```python
from build123d import *

# Parameters (mm, degrees)
F0_W     = 183.4
F0_H     = 218.4
F1_DEPTH = 49.6
F2_T     = -1.2
F3_R     = 2
F4_R     = 0.8


with BuildPart() as f1:
    # F0 (on Top) → F1 (new body)
    with BuildSketch(Plane.XY):
        Rectangle(F0_W, F0_H)
    extrude(amount=F1_DEPTH)

    # F2
    f2_openings = [f1.faces().sort_by_distance(p)[0] for p in [
        (0, 0, 0),
    ]]
    offset(amount=F2_T, openings=f2_openings)

    # F3
    f3_edges = [f1.edges().sort_by_distance(p)[0] for p in [
        (-91.7, -109.2, 24.8),
        (-91.7, 109.2, 24.8),
        (91.7, 109.2, 24.8),
        (91.7, -109.2, 24.8),
    ]]
    fillet(f3_edges, radius=F3_R)

    # F4
    f4_edges = [f1.edges().sort_by_distance(p)[0] for p in [
        (-90.5, -108, 24.2),
        (90.5, -108, 24.2),
        (90.5, 108, 24.2),
        (-90.5, 108, 24.2),
    ]]
    fillet(f4_edges, radius=F4_R)


solid = f1.part
```
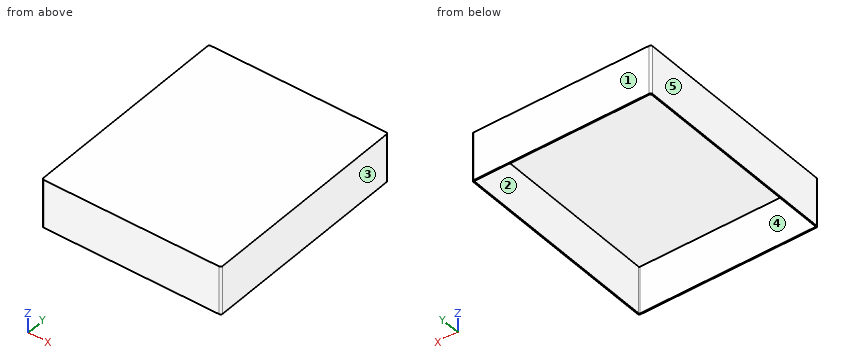
The listing builds one solid part. Answer for the finished solid, in the listing's coordinates (mm). Face numbers are marked on the shaded views. A direction names the side the tool comes from. Coordinates: 2 decimals unless noted, no trailing zeros. Write each loop counter-clockwise with the first axis right and the second up, starting at its lowest first coordinate (ties: lowest second). Pieces come first, ordered by that corner, then holes. Notation, with made-up numbers: (66.5, 40) - (93.5, 40) arc R21 cw to (93.5, 67) - close; hole circle Ø10 at (56, 8.25). An arc over 180 degrees is marked (long way). One line per item, written item: value.
1) For a pull along X with two mould halves and no side action, classify the marked faces 3, 4 and 5 as pulls with the +X half, pulls with the -X half, needs draft (parallel to the pull), parting line crosses it, or undercut.
Geometry check:
face 3: pulls with the +X half
face 4: undercut
face 5: pulls with the -X half
2) Find section A-A (z = 24). Give the vertices of the cut face in (x, y).
Geometry check:
outline: (-91.7, -107.2) arc R2 ccw to (-89.7, -109.2) - (89.7, -109.2) arc R2 ccw to (91.7, -107.2) - (91.7, 107.2) arc R2 ccw to (89.7, 109.2) - (-89.7, 109.2) arc R2 ccw to (-91.7, 107.2) - close; hole (-90.5, -107.2) arc R0.8 ccw to (-89.7, -108) - (89.7, -108) arc R0.8 ccw to (90.5, -107.2) - (90.5, 107.2) arc R0.8 ccw to (89.7, 108) - (-89.7, 108) arc R0.8 ccw to (-90.5, 107.2) - close
3) Find section B-B (x = 4.5). Give the vertices of the cut face in (y, z).
Geometry check:
outline: (-109.2, 0) - (-108, 0) - (-108, 48.4) - (108, 48.4) - (108, 0) - (109.2, 0) - (109.2, 49.6) - (-109.2, 49.6) - close
4) Consider line 1 along Y through (x, z) = (-67.5, 22); line 2 along X through (y, z) = (-93, 44.5); line 3 along Z through (x, y) = (7, 12.5). Determine where each line is inside the solid, lowest interval first. Write a range as from..to.
Geometry check:
line 1: y = -109.2..-108, 108..109.2
line 2: x = -91.7..-90.5, 90.5..91.7
line 3: z = 48.4..49.6
5) A tool of negligible diameter and unlimited length cuts with its end or side. For the marked faces 1 and 2, from which of +Z, -Z, +X, -X, +Y, -Y can it reach the whole face along a straight path? Write none if from no direction.
Geometry check:
face 1: +Z, -Z, +X, -X, +Y
face 2: -Z
6) Find section C-C (y = 94.5). Give the vertices of the cut face in (x, z), and give its area (3 significant figures).
Geometry check:
outline: (-91.7, 0) - (-90.5, 0) - (-90.5, 48.4) - (90.5, 48.4) - (90.5, 0) - (91.7, 0) - (91.7, 49.6) - (-91.7, 49.6) - close
area: 336 mm2
7) This flat-tipped pin is pushed along its axis until it touches: pin 1 Ø12 at (x, y) = (-32.5, 44) entering from -Z. Where does it stop, or does it pass through?
Geometry check:
pin 1: stops at z = 48.4
